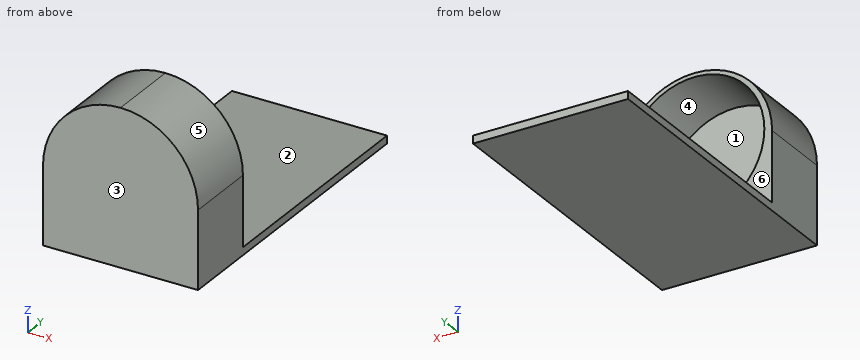
```python
from build123d import *

# Parameters (mm, degrees)
F0_W     = 40
F0_H     = 61
F1_DEPTH = 2
F0_H_2   = 19
F2_DEPTH = 40
F3_R     = 18
F4_DEPTH = 17
F5_R     = 19.99999


# Not quite as in the source:
# - a fillet or chamfer is up to 0.001 mm smaller than in the source, because OpenCascade refuses the exact size


with BuildPart() as f1:
    # F0 (on Top) → F1 (new body)
    with BuildSketch(Plane.XY):
        with Locations((-2.8480109572, 28.6193176061)):
            Rectangle(F0_W, F0_H)
    extrude(amount=F1_DEPTH)

    # F0 (on Top) → F2 (join)
    with BuildSketch(Plane.XY):
        with Locations((-2.8480109572, -11.3806823939)):
            Rectangle(F0_W, F0_H_2)
    extrude(amount=F2_DEPTH)

    # F3 (on face) → F4 (cut)
    with BuildSketch(Plane(origin=(0, -1.8806823939, 0), x_dir=(-1, 0, 0), z_dir=(0, 1, 0))):
        with Locations((2.8480109572, 21)):
            Circle(F3_R)
    extrude(amount=-F4_DEPTH, mode=Mode.SUBTRACT)

    # F5 (radius 20 in the source; OpenCascade refuses exactly that, so slightly less here)
    f5_edges = [f1.edges().sort_by_distance(p)[0] for p in [
        (17.151989, -11.380682, 40),
        (-22.848011, -11.380682, 40),
    ]]
    fillet(f5_edges, radius=F5_R)


solid = f1.part
```
Part model, mm, in its own coordinate system. Face numbers are marked on the shaded views. A direction names the side the tool comes from. Round coordinates to 2 decimals unless told otherwise and drop trailing zeros. Loops run counter-clockwise (first coordinate to the right, second up) from the corner with the lowest first, then second, coordinate; pieces in that order, holes last.
Item 1: 3-axis set-ups, long thin cutter, end or side, ignore diameter. For the marked faces 1, 2 and 3: which of +Z, -Z, +X, -X, +Y, -Y reach the whole face in a straight line?
Item 2: Cut at D-D, the plane z = 21. Give the cut face in (x, y), then the cut area to 3 significant figures.
Item 3: Cut at C-C, the plane x = -16.5. Give the cut face in (y, z), then the cut area to 3 significant figures.
Item 4: Drop flat-ended pins along their axis: P1, Ø11.5, axis at x = 5, z = 15.5, coming from the +Y side; P2, Ø1.5, axis at x = -12, y = 23.5, coming from the +Z side. Give the stop position or say it passes through.
Item 5: Mould opens along Z. For the marked faces 4, 5 and 6 say: +Z half, -Z half, draft (parallel to the pull), parting line (faces both ways), or undercut.
Item 6: Cut at B-B, the plane z = 7.5. Give the cut face in (x, y).
Item 7: Drill centre lines: line 1 (Y direction, x = -4, z = 18); line 2 (Z direction, x = -8.5, y = 6.5); line 3 (Y direction, x = -17.5, z = 3.5). Where is each one in solid material? Low to high.
A:
1. face 1: +Y
1. face 2: +Z, +X, -X, +Y
1. face 3: +Z, -Z, +X, -X, -Y
2. outline: (-22.82, -20.88) - (17.13, -20.88) - (17.13, -1.88) - (15.15, -1.88) - (15.15, -18.88) - (-20.85, -18.88) - (-20.85, -1.88) - (-22.82, -1.88) - close
2. area: 147 mm2
3. outline: (-20.88, 0) - (59.12, 0) - (59.12, 2) - (-1.88, 2) - (-1.88, 9.27) - (-18.88, 9.27) - (-18.88, 32.73) - (-1.88, 32.73) - (-1.88, 34.62) - (-20.88, 34.62) - close
3. area: 381 mm2
4. P1: stops at y = -18.88
4. P2: stops at z = 2
5. face 4: undercut
5. face 5: +Z half
5. face 6: draft
6. outline: (-22.85, -20.88) - (17.15, -20.88) - (17.15, -1.88) - (9.06, -1.88) - (9.06, -18.88) - (-14.75, -18.88) - (-14.75, -1.88) - (-22.85, -1.88) - close
7. line 1: y = -20.88 to -18.88
7. line 2: z = 0 to 2
7. line 3: y = -20.88 to -1.88
